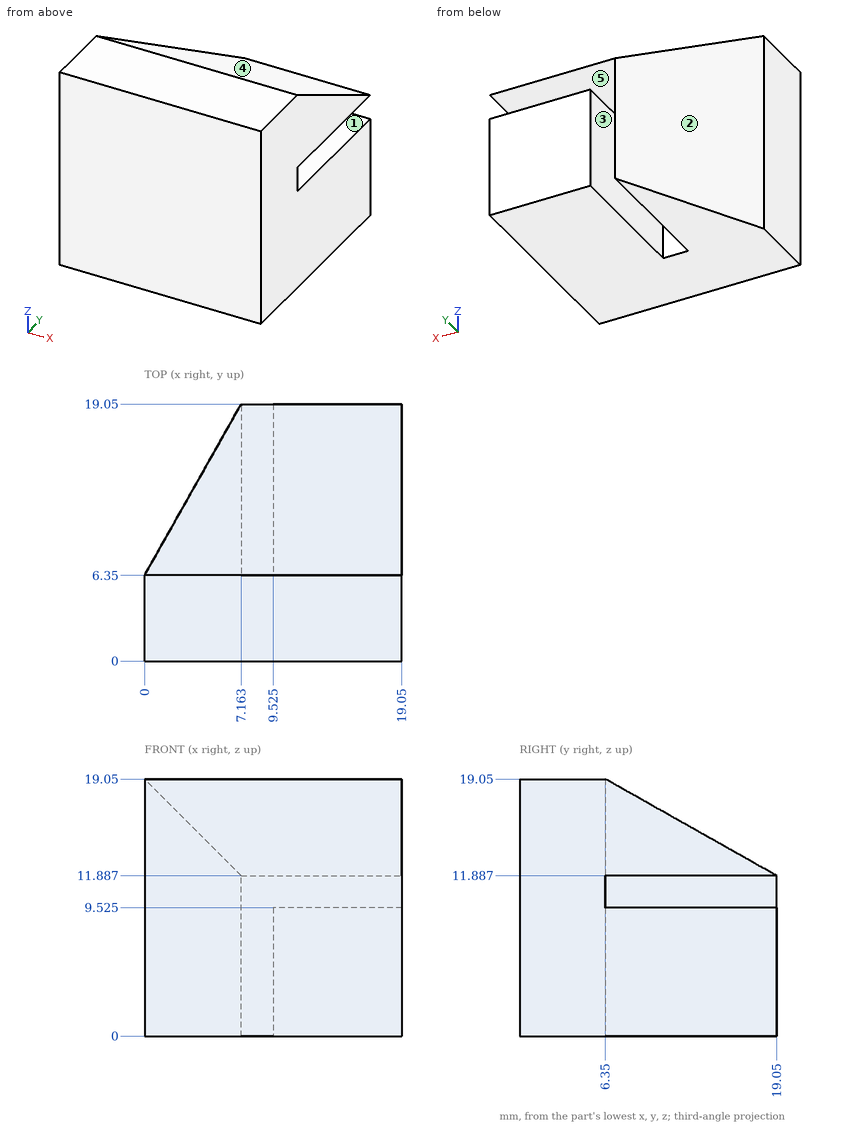
Input: dimensioned drawing with shaded views. Units: mm. Origin: part minimum x, y, z. A direction names the side the tool comes from. Round coordinates to 2 decimals unless told otherwise and drop trailing zeros. Use one line per item in the form item = value. Start each with the question number.
Q1. Material intervals for line 1 (Y direction, x = 14, z = 11.5); line 2 (Z direction, x = 13.25, y = 13.5) (1 decimal); line 3 (Z direction, x = 11, y = 8.25) (1 decimal), sorted ascending. Write a range as [from, to].
Q2. Pin query (flat end, axial travel): pin 1 Ø6 at (y, z) = (12, 5.5) entering from -X (1 decimal); pin 2 Ø5 at (y, z) = (12, 5) entering from -X; pin 3 Ø4 at (y, z) = (12, 15) entering from -X. Return the tip coordinate at first contact, or that it passes through.
Q3. Mould query, pull axis Z, two halves, no side actions, for the marked faces 3, 4 and 5. Classes: +Z half, -Z half, draft (parallel to the pull), parting line (faces both ways), or undercut.
Q4. Access query for the marked faces 1 and 2. Directions: +Z, -Z, +X, -X, +Y, -Y. A direction counts if a zero-diameter tool reaches every point of the face in a straight line with its end or side. Return the directions, or none.
Geometry results:
q1.line_1 = [0, 6.35]
q1.line_2 = [0, 9.5], [11.9, 15]
q1.line_3 = [0, 9.5], [11.9, 18]
q2.pin_1 = 1.5
q2.pin_2 = 1.78
q2.pin_3 = 2.06
q3.face_3 = draft
q3.face_4 = +Z half
q3.face_5 = undercut
q4.face_1 = +X, +Y
q4.face_2 = +Z, -Z, -X, +Y
